The drawing under review shows one solid part. Ordinate dimensions are in mm from its lowest x, y, z. A direction names the side the tool comes from. Round coordinates to 2 decimals unless told otherwise and drop trailing zeros. Write each loop counter-clockwise with the first axis right and the second up, starting at its lowest first coordinate (ties: lowest second). Pieces come first, ordered by that corner, then holes. Notation, with made-up numbers: M -27.5,60.25 L 5.5,60.25 A24 cw 5.5,71.25 Z; hole C 82,-12.5 d7. An arc over 180 degrees is marked long. Write item = value, one per line. Start each with the question number.
Item 1: Take a section at C-C, the plane z = 19.25. Give the boundary of the cut face in (x, y).
Item 2: Take a section at B-B, the plane x = 11. Give the boundary of the cut face in (y, z), plus the area to 3 significant figures.
Item 3: For pin 1 Ø2 at (x, y) = (10, 19.5) entering from +Z; pin 2 Ø12 at (x, z) = (7.5, 16) entering from -Y; pin 3 Ø1.6 at (x, y) = (2.5, 20.5) entering from +Z, all flat-tipped, find the tip position at first contact; note any pin that passes through.
Item 4: Tool access review of the marked faces 1, 2 and 3: name each direction out of +Z, -Z, +X, -X, +Y, -Y from which nothing blocks a thin tool from reaching the whole face with its end or side.
Item 5: Take a section at D-D, the plane x = 18. Give the boundary of the cut face in (y, z).
Item 6: To check wall thickness, follow line 1 along Z through (x, y) = (11.25, 7); line 2 along Y through (x, z) = (6.25, 10.5); line 3 along Y through (x, z) = (17.25, 8.5). State the ranges of each line that lie inside material, in increasing order.
Item 7: Take a section at A-A, the plane y = 22.5. Give the boundary of the cut face in (x, z).
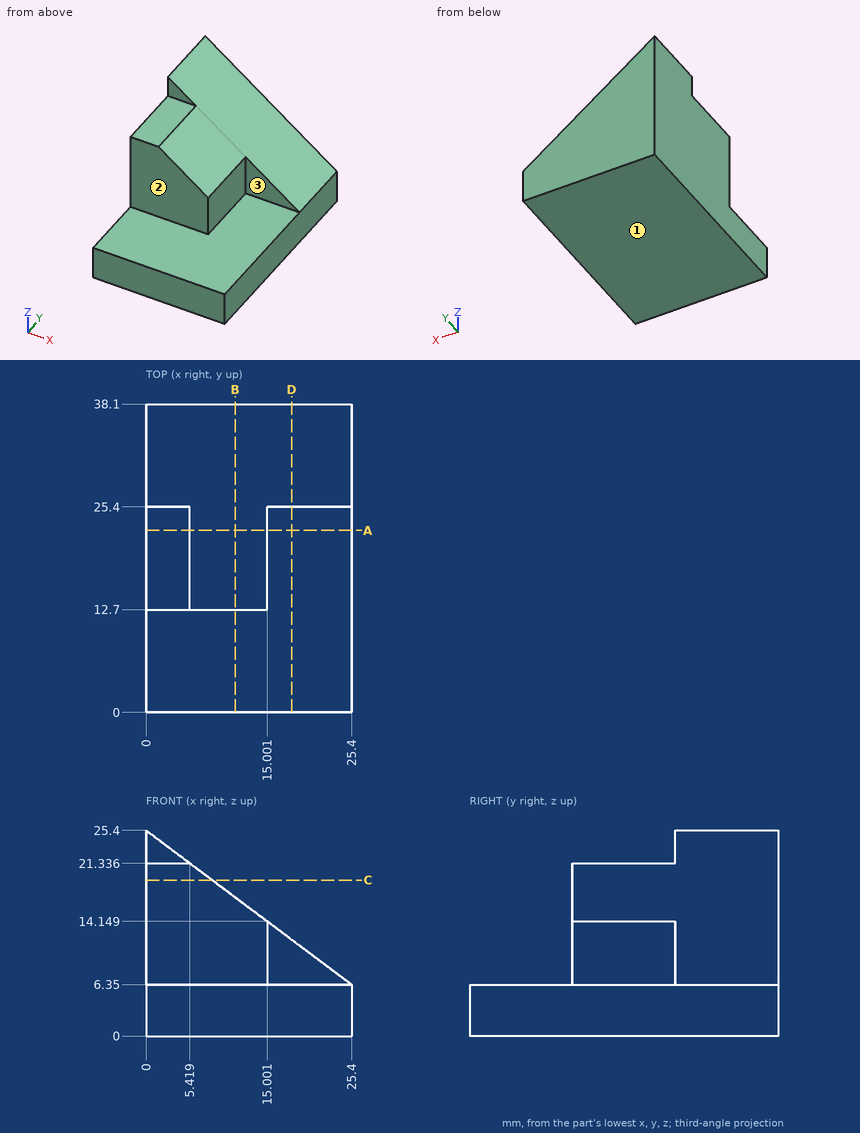
Response values:
q1.outline = M 0,12.7 L 8.2,12.7 L 8.2,38.1 L 0,38.1 Z
q2.outline = M 0,0 L 38.1,0 L 38.1,17.15 L 12.7,17.15 L 12.7,6.35 L 0,6.35 Z
q2.area = 516 mm2
q3.pin_1 = 18.65
q3.pin_2 = 12.7
q3.pin_3 = 21.34
q4.face_1 = -Z, +X, -X, +Y, -Y
q4.face_2 = +Z, +X, -X, -Y
q4.face_3 = +Z, +X, -Y
q5.outline = M 0,0 L 38.1,0 L 38.1,11.9 L 25.4,11.9 L 25.4,6.35 L 0,6.35 Z
q6.line_1 = 0 to 6.35
q6.line_2 = 12.7 to 38.1
q6.line_3 = 25.4 to 38.1
q7.outline = M 0,0 L 25.4,0 L 25.4,6.35 L 15,6.35 L 15,14.15 L 5.42,21.34 L 0,21.34 Z
